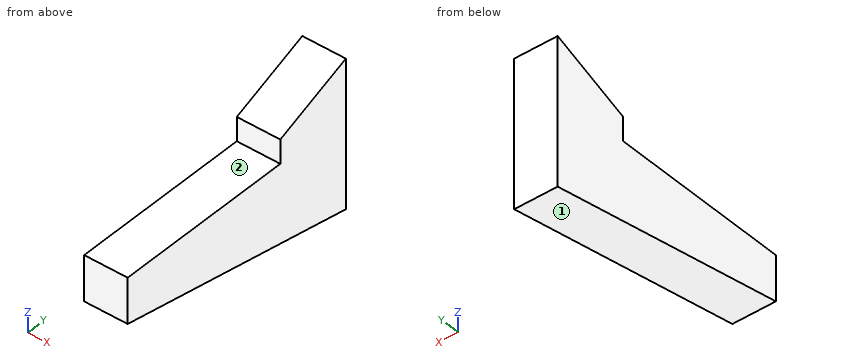
```python
from build123d import *

# Parameters (mm, degrees)
F1_DEPTH = 25.4


with BuildPart() as f1:
    # F0 (on Right) → F1 (new body)
    with BuildSketch(Plane.YZ):
        Polygon((16.642717, 0), (-75.669996, 0), (-75.669996, -26.522875), (76.867461, -54.014966), (76.867461, -26.522875), (31.040281, 0), (25.836868, 0), (29.329389, -22.730291), align=None)
        Polygon((25.836868, 0), (16.642717, 0), (29.329389, -22.730291), align=None)
        Polygon((31.040281, 13.931453), (31.040281, 0), (76.867461, -26.522875), (76.867461, 32.262325), align=None)
    extrude(amount=F1_DEPTH)


solid = f1.part
```
Work out the finished part from the listing and answer in its coordinate system (mm). Face numbers are marked on the shaded views. A direction names the side the tool comes from. Give positions to 0.01 mm unless a question says otherwise; leave off trailing zeros. Order: outer loops, then holes, each group sorted by start corner. A loop starts at its lowest first (then second) coordinate and runs counter-clockwise, first axis right, second up.
1. Straight lines are drawn through the part: L1, parallel to Y at x = 24, z = 12.5; L2, parallel to Z at x = 18.5, y = 2; L3, parallel to Z at x = 20.5, y = -30.5. For each, find the intervals that lie inside material, in ascending order.
Result sheet:
L1: y = 31.04 to 76.87
L2: z = -40.52 to 0
L3: z = -34.66 to 0
2. For the marked faces 1 and 2, determine the directions among +Z, -Z, +X, -X, +Y, -Y from which every point of the face is accessible in a straight line to the end or side of a thin tool.
Result sheet:
face 1: -Z, +X, -X, -Y
face 2: +Z, +X, -X, -Y
3. Section B-B, the plane z = 11 is taken. Determine the outline of the cut face in (x, y).
Result sheet:
outline: (0, 31.04) - (25.4, 31.04) - (25.4, 76.87) - (0, 76.87) - close
4. Each of these flat-tipped pins is pushed along its axis until it touches: P1, Ø7.5, axis at x = 9, y = -33.5, coming from the +Z side; P2, Ø7, axis at x = 7, z = 4, coming from the -Y side. Where does it stop, or does it pass through?
Result sheet:
P1: stops at z = 0
P2: stops at y = 31.04
5. Section C-C, the plane y = -49 is taken. Determine the outline of the cut face in (x, z), and give its area (3 significant figures).
Result sheet:
outline: (0, -31.33) - (25.4, -31.33) - (25.4, 0) - (0, 0) - close
area: 796 mm2
6. Section A-A, the plane x = 17.5 is taken. Determine the outline of the cut face in (y, z).
Result sheet:
outline: (-75.67, -26.52) - (76.87, -54.01) - (76.87, 32.26) - (31.04, 13.93) - (31.04, 0) - (-75.67, 0) - close
